Model file for the job. Use its own axes, mm. A direction names the side the tool comes from. Coordinates: 2 decimals unless noted, no trailing zeros. Write each loop counter-clockwise with the first axis right and the second up, starting at its lowest first coordinate (ties: lowest second). Pieces come first, ordered by that corner, then holes. Notation, with made-up numbers: (-8, 67.25) -> (-3, 67.25) arc R25 ccw to (-3, 99.25) -> close; hole circle Ø7 at (62, 69.25). An arc over 180 degrees is marked (long way). Answer as a JSON object with one key per item and string values. Group by question number.
from build123d import *

# Parameters (mm, degrees)
CROQUIS1_R              = 11.25
CROQUIS1_R_2            = 2
SALIENTE_EXTRUIR2_DEPTH = 2.5
CROQUIS2_R              = 12.5
CROQUIS2_R_2            = 11.25
SALIENTE_EXTRUIR4_DEPTH = 80
REDONDEO1_R             = 1


with BuildPart() as part:
    # Croquis1 → Saliente-Extruir2 (new body)
    with BuildSketch(Plane(origin=(0, 0, 0), x_dir=(1, 0, 0), z_dir=(0, 1, 0))):
        with BuildLine():
            Line((-17.5, 6), (-16.439282223, 6))
            ThreePointArc((-16.439282223, 6), (0, 17.5), (16.439282223, 6))
            Line((16.439282223, 6), (17.5, 6))
            ThreePointArc((17.5, 6), (23.5, 0), (17.5, -6))
            Line((17.5, -6), (16.439282223, -6))
            ThreePointArc((16.439282223, -6), (0, -17.5), (-16.439282223, -6))
            Line((-16.439282223, -6), (-17.5, -6))
            ThreePointArc((-17.5, -6), (-23.5, 0), (-17.5, 6))
        make_face()
        with Locations(Location((0, 0, 0), (0, 0, 270))):
            Circle(CROQUIS1_R, mode=Mode.SUBTRACT)
        with Locations(Location((-17.5, 0, 0), (0, 0, 270))):
            Circle(CROQUIS1_R_2, mode=Mode.SUBTRACT)
        with Locations(Location((17.5, 0, 0), (0, 0, 270))):
            Circle(CROQUIS1_R_2, mode=Mode.SUBTRACT)
    extrude(amount=SALIENTE_EXTRUIR2_DEPTH)

    # Croquis2 → Saliente-Extruir4 (add)
    with BuildSketch(Plane(origin=(0, 2.5, 0), x_dir=(1, 0, 0), z_dir=(0, 1, 0))):
        with Locations(Location((0, 0, 0), (0, 0, 270))):
            Circle(CROQUIS2_R)
        with Locations(Location((0, 0, 0), (0, 0, 270))):
            Circle(CROQUIS2_R_2, mode=Mode.SUBTRACT)
    extrude(amount=SALIENTE_EXTRUIR4_DEPTH)

    # Redondeo1
    redondeo1_edges = [part.edges().sort_by_distance(p)[0] for p in [
        (16.969641111, 0, 6),
        (0, 0, 17.5),
        (-16.969641111, 0, 6),
        (-23.5, 0, 0),
        (0, 0, -11.25),
        (-16.969641111, 0, -6),
        (0, 0, -17.5),
        (16.969641111, 0, -6),
        (23.5, 0, 0),
    ]]
    fillet(redondeo1_edges, radius=REDONDEO1_R)


solid = part.part
(1) Cut at B-B on z = 0. List the corners of the cut face in (x, y).
(2) Cut at C-C on y = 24. List the corners of the cut face in (x, z).
(3) 3-axis set-ups, long thin cutter, end or side, ignore diameter. For faces 1 (the face through (12, 0, -4)), 2 (the face through (3.755, 41.94, 11.923)): which of +Z, -Z, +X, -X, +Y, -Y reach the whole face in a straight line?
(4) Pull direction X, two halves, no side cores. Call faces 3 (the face through (-23.5, 1.7, 0.1)), 4 (the face through (-4.31, 41.18, 10.39)), 5 (the face through (0.299, 1.739, 17.497)), 6 (the face through (-10, 2.5, -8)): released by +X, released by -X, zero draft, split by the parting line, or undercut.
(5) Wall check: probe 1 along X at (y, z) = (1, 0); probe 2 along X at (y, z) = (34, 0); probe 3 along Y at (x, z) = (-19, 4.5). Give the ranges that are in metal, low to high.
(6) Pin check, flat tips, straight feed: pin 1 (0.8 mm diameter, centred on x = -17, y = 1.5, fed in from +Z); pin 2 (5 mm diameter, centred on x = 17.5, z = 0, fed in from +Y); pin 3 (3 mm diameter, centred on y = 34.5, z = 7.5, fed in from -X); pin 4 (3 mm diameter, centred on x = 13, z = 5, fed in from +Y). Stop position of each tip, or through.
(7) Cut at A-A on x = 0. List the corners of the cut face in (y, z), plus the area to 3 significant figures.
Results found:
{
 "1": {"outline": "(-23.5, 1) arc R1 ccw to (-22.5, 0) -> (-19.5, 0) -> (-19.5, 2.5) -> (-23.5, 2.5) -> close; (-15.5, 0) -> (-12.25, 0) arc R1 ccw to (-11.25, 1) -> (-11.25, 82.5) -> (-12.5, 82.5) -> (-12.5, 2.5) -> (-15.5, 2.5) -> close; (11.25, 1) arc R1 ccw to (12.25, 0) -> (15.5, 0) -> (15.5, 2.5) -> (12.5, 2.5) -> (12.5, 82.5) -> (11.25, 82.5) -> close; (19.5, 0) -> (22.5, 0) arc R1 ccw to (23.5, 1) -> (23.5, 2.5) -> (19.5, 2.5) -> close"},
 "2": {"outline": "circle Ø25 at (0, 0); hole circle Ø22.5 at (0, 0)"},
 "3": {"face 1": "+Z, -Z, +X, -X, -Y", "face 2": "+Y"},
 "4": {"face 3": "released by -X", "face 4": "undercut", "face 5": "split by the parting line", "face 6": "zero draft"},
 "5": {"probe 1": "x = -23.5 to -19.5, -15.5 to -11.25, 11.25 to 15.5, 19.5 to 23.5", "probe 2": "x = -12.5 to -11.25, 11.25 to 12.5", "probe 3": "y = 0 to 2.5"},
 "6": {"pin 1": "stops at z = 6", "pin 2": "stops at y = 2.5", "pin 3": "stops at x = -10.97", "pin 4": "stops at y = 82.5"},
 "7": {"outline": "(0, -16.5) arc R1 ccw to (1, -17.5) -> (2.5, -17.5) -> (2.5, -12.5) -> (82.5, -12.5) -> (82.5, -11.25) -> (1, -11.25) arc R1 ccw to (0, -12.25) -> close; (0, 12.25) arc R1 ccw to (1, 11.25) -> (82.5, 11.25) -> (82.5, 12.5) -> (2.5, 12.5) -> (2.5, 17.5) -> (1, 17.5) arc R1 ccw to (0, 16.5) -> close", "area": "230 mm²"}
}
